```python
from build123d import *

# Parameters (mm, degrees)
F1_DEPTH = 7.5
F3_D     = 3.3
F5_D     = 3.3


with BuildPart() as f1:
    # F0 (on Front) → F1 (new body, symmetric)
    with BuildSketch(Plane.XZ):
        Polygon((0, -2), (0, 0), (-8, 0), (-8, 2.5), (-20, 2.5), (-20, 0.5), (-10, 0.5), (-10, -2), align=None)
    extrude(amount=F1_DEPTH, both=True)

    # F3 (through all)
    with Locations(Plane.XY.offset(2.5)):
        with Locations((-15, -3.5), (-15, 3.5)):
            Hole(F3_D / 2)

    # F5 (through all)
    with Locations(Plane.XY):
        with Locations((-4, -5), (-4, 5)):
            Hole(F5_D / 2)


solid = f1.part
```
Geometry: final body of the model. Coordinates: model frame, mm. A direction names the side the tool comes from. Coordinates: 2 decimals unless noted, no trailing zeros. Order: outer loops, then holes, each group sorted by start corner. A loop starts at its lowest first (then second) coordinate and runs counter-clockwise, first axis right, second up. Notation, with made-up numbers: M 4.25,9 L 50.25,9 A22 ccw 50.25,24 Z; hole C 37.5,58 d7. An arc over 180 degrees is marked long. Answer in a Markdown table with one row per item. Add a question column.
Q1. Line query: L1, parallel to Y at x = -4, z = -1.5; L2, parallel to Y at x = -15, z = 1.8; L3, parallel to X at y = 1.75, z = -0.9. Output: solid intervals per line, ascending.
Q2. Mould query, pull axis Y, two halves, no side actions, for faces 4 (the flat face through (-10, -7.5, 1)), 5 (the cylindrical face through (-16.574, -3.004, 1.486)), 6 (the flat face through (-10, 7.5, 1)), 7 (the flat face through (-14, 0, 2.5)). Classes: released by +Y, released by -Y, zero draft, split by the parting line, or undercut.
Q3. Section query B-B on y = 0.25. Return the cut outline in (x, z), and give its area (3 significant figures).
Q4. Section query C-C on z = -0.8. Return the cut outline in (x, y), and give its area (3 significant figures).
Q5. Reachability of faces 1 (the flat face through (-10, 0, -1)), 2 (the flat face through (-8, 0, 1)), 3 (the flat face through (-20, 0, 2)) from +Z, -Z, +X, -X, +Y, -Y: full face, straight path, thin tool, end or side. Return the list, or none.
Q6. Contact query for flat-ended pins moving along their axis: P1, Ø2.5, axis at x = -4, y = 5, coming from the -Z side; P2, Ø2, axis at x = -15.5, y = -4, coming from the -Z side; P3, Ø4, axis at x = -3.5, y = -3, coming from the +Z side; P4, Ø1.2, axis at y = -1, z = 1.5, coming from the +X side. Output: stop coordinate, or through.
Q7. Section query D-D on y = 3. Return the cut outline in (x, z), and give its area (3 significant figures).
Q8. Section query A-A on x = -15. Return the cut outline in (y, z), and give its area (3 significant figures).
Completed:
| question | item | result |
|---|---|---|
| 1 | L1 | y = -7.5 to -6.65, -3.35 to 3.35, 6.65 to 7.5 |
| 1 | L2 | y = -7.5 to -5.15, -1.85 to 1.85, 5.15 to 7.5 |
| 1 | L3 | x = -10 to 0 |
| 2 | face 4 | released by -Y |
| 2 | face 5 | undercut |
| 2 | face 6 | released by +Y |
| 2 | face 7 | zero draft |
| 3 | outline | M -20,0.5 L -10,0.5 L -10,-2 L 0,-2 L 0,0 L -8,0 L -8,2.5 L -20,2.5 Z |
| 3 | area | 45.0 mm2 |
| 4 | outline | M -10,-7.5 L 0,-7.5 L 0,7.5 L -10,7.5 Z; hole C -4,-5 d3.3; hole C -4,5 d3.3 |
| 4 | area | 133 mm2 |
| 5 | face 1 | -Z, -X, +Y, -Y |
| 5 | face 2 | +Z, +X, +Y, -Y |
| 5 | face 3 | +Z, -Z, -X, +Y, -Y |
| 6 | P1 | passes through |
| 6 | P2 | stops at z = 0.5 |
| 6 | P3 | stops at z = 0 |
| 6 | P4 | stops at x = -8 |
| 7 | outline | M -20,0.5 L -16.57,0.5 L -16.57,2.5 L -20,2.5 Z; M -13.43,0.5 L -10,0.5 L -10,-2 L 0,-2 L 0,0 L -8,0 L -8,2.5 L -13.43,2.5 Z |
| 7 | area | 38.7 mm2 |
| 8 | outline | M -7.5,0.5 L -5.15,0.5 L -5.15,2.5 L -7.5,2.5 Z; M -1.85,0.5 L 1.85,0.5 L 1.85,2.5 L -1.85,2.5 Z; M 5.15,0.5 L 7.5,0.5 L 7.5,2.5 L 5.15,2.5 Z |
| 8 | area | 16.8 mm2 |
